Drawing for the job (mm, zero at the part's lowest x, y, z). A direction names the side the tool comes from. Give positions to 0.01 mm unless a question says otherwise; leave off trailing zeros. Loops run counter-clockwise (first coordinate to the right, second up) from the corner with the lowest first, then second, coordinate; pieces in that order, holes last. Notation, with made-up numbers: (57.5, -17.5) -> (81.5, -17.5) arc R34 ccw to (81.5, 13.5) -> close; hole circle Ø5 at (-5.5, 8). An arc over 180 degrees is marked (long way). Write item = value, one per line.
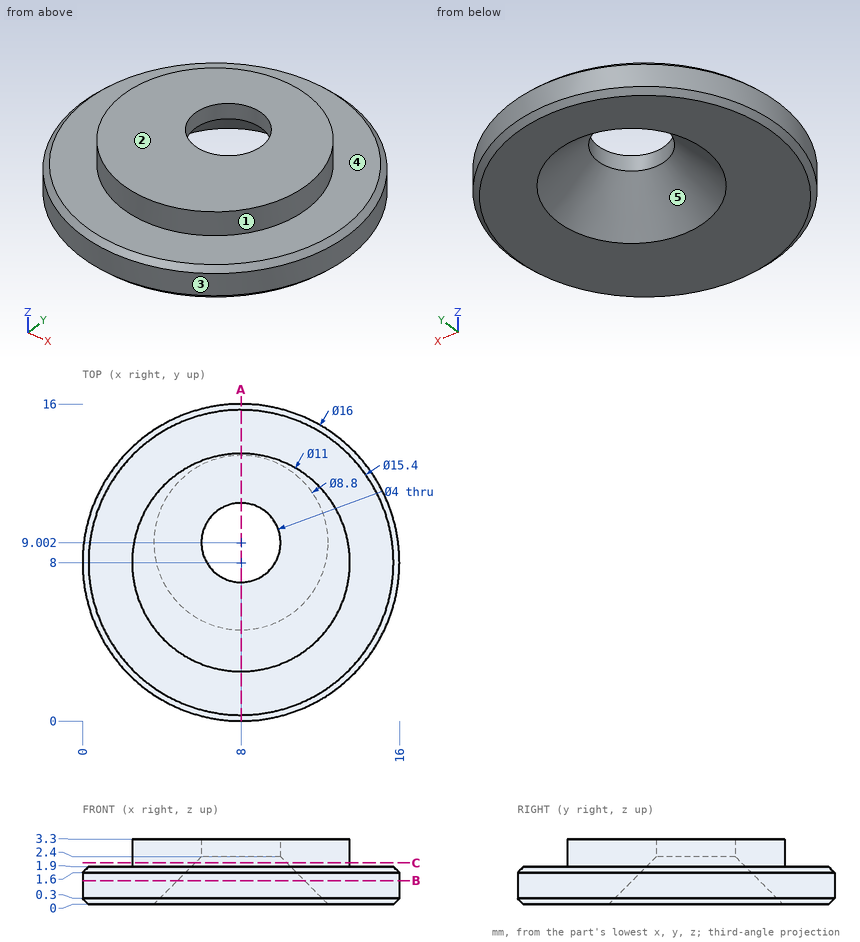
1) Slice it at C-C, the plane z = 2.1. List the corners of the cut face in (x, y).
Resolved:
outline = circle Ø11 at (8, 8); hole circle Ø4.6 at (8, 9)
2) Slice it at A-A, the plane x = 8. List the corners of the cut face in (y, z).
Resolved:
outline = (0, 0.3) -> (0.3, 0) -> (4.6, 0) -> (7, 2.4) -> (7, 3.3) -> (2.5, 3.3) -> (2.5, 1.9) -> (0.3, 1.9) -> (0, 1.6) -> close; (11, 2.4) -> (13.4, 0) -> (15.7, 0) -> (16, 0.3) -> (16, 1.6) -> (15.7, 1.9) -> (13.5, 1.9) -> (13.5, 3.3) -> (11, 3.3) -> close
3) Drop a flat-ended pin along its axis: P1, Ø1, axis at x = 5, z = 1.5, coming from the +Y side. Give the stop position or say it passes through.
Resolved:
P1 = 15.6
4) Drill centre lines: line 1 along Y through (x, z) = (8, 2.65); line 2 along X through (y, z) = (6.75, 0.9); line 3 along Y through (x, z) = (4.75, 0.5) (1 decimal). Where is each one in solid material? Low to high. Write a range as [from, to].
Resolved:
line_1 = [2.5, 7], [11, 13.5]
line_2 = [0.1, 5.32], [10.68, 15.9]
line_3 = [0.7, 6.8], [11.2, 15.3]
5) Pull direction X, two halves, no side cores. Call the marked faces 3, 4 and 5: pulls with the +X half, pulls with the -X half, needs draft (parallel to the pull), parting line crosses it, or undercut.
Resolved:
face_3 = parting line crosses it
face_4 = needs draft
face_5 = undercut
6) Slice it at B-B, the plane z = 1.2. List the corners of the cut face in (x, y).
Resolved:
outline = circle Ø16 at (8, 8); hole circle Ø6.4 at (8, 9)
7) Which spindle directions (+Z, -Z, +X, -X, +Y, -Y) get a long thin tool onto all of the face, cutting with end or side? Do the marked faces 1 and 2. Say none if no direction does.
Resolved:
face_1 = +Z
face_2 = +Z, +X, -X, +Y, -Y
